Geometry check sheet. Reference: the model listing, model coordinates, mm. Give positions to 0.01 mm unless a question says otherwise; leave off trailing zeros. Loops run counter-clockwise (first coordinate to the right, second up) from the corner with the lowest first, then second, coordinate; pieces in that order, holes last. Notation, with made-up numbers: (41, -19) -> (63, -19) arc R18 cw to (63, -5) -> close; hole circle Ø8 at (36, 7.5). An arc over 180 degrees is marked (long way). Answer as a JSON object with one key per item and string values.
from build123d import *

# Parameters (mm, degrees)
SKETCH1_W           = 228.6
SKETCH1_H           = 228.6
BOSS_EXTRUDE1_DEPTH = 5.08
CUT_EXTRUDE2_REACH  = 325.329
SKETCH9_W           = 5.08
SKETCH9_H           = 12.7
SKETCH9_H_2         = 50.8
CUT_EXTRUDE7_START  = -5.08
CUT_EXTRUDE7_DEPTH  = 5.08
CUT_EXTRUDE5_REACH  = 325.329
SKETCH13_R          = 1.7
CUT_EXTRUDE6_REACH  = 325.329
SKETCH16_W          = 5.08
SKETCH16_H          = 12.7
CUT_EXTRUDE8_DEPTH  = 324.329130287
SKETCH17_W          = 20.32
SKETCH17_H          = 5.08
CUT_EXTRUDE9_DEPTH  = 324.329130287
CUT_EXTRUDE10_REACH = 325.329
SKETCH18_R          = 31.75
CUT_EXTRUDE11_REACH = 325.329
SKETCH19_W          = 20.828
SKETCH19_H          = 12.065


# Read off the part's stored shape, not the designer's step: Cut-Extrude7
with BuildPart() as part:
    # Sketch1 → Boss-Extrude1 (new body)
    with BuildSketch(Plane(origin=(0, 0, 0), x_dir=(1, 0, 0), z_dir=(0, 1, 0))):
        with Locations((114.3, 114.3)):
            Rectangle(SKETCH1_W, SKETCH1_H)
    extrude(amount=BOSS_EXTRUDE1_DEPTH)

    # Sketch9 → Cut-Extrude2 (cut, up to next)
    with BuildSketch(Plane(origin=(0, 5.08, 0), x_dir=(1, 0, 0), z_dir=(0, 1, 0)), mode=Mode.PRIVATE) as cut_extrude2_sk1:
        with Locations((27.94, 57.15)):
            Rectangle(SKETCH9_W, SKETCH9_H)
    cut_extrude2_tool1 = extrude(cut_extrude2_sk1.sketch, amount=-CUT_EXTRUDE2_REACH, mode=Mode.PRIVATE) & part.part
    # Sketch9 → Cut-Extrude2 (cut, up to next)
    with BuildSketch(Plane(origin=(0, 5.08, 0), x_dir=(1, 0, 0), z_dir=(0, 1, 0)), mode=Mode.PRIVATE) as cut_extrude2_sk2:
        with Locations((27.94, 171.45)):
            Rectangle(SKETCH9_W, SKETCH9_H)
    cut_extrude2_tool2 = extrude(cut_extrude2_sk2.sketch, amount=-CUT_EXTRUDE2_REACH, mode=Mode.PRIVATE) & part.part
    # Sketch9 → Cut-Extrude2 (cut, up to next)
    with BuildSketch(Plane(origin=(0, 5.08, 0), x_dir=(1, 0, 0), z_dir=(0, 1, 0)), mode=Mode.PRIVATE) as cut_extrude2_sk3:
        with Locations((27.94, 114.3)):
            Rectangle(SKETCH9_W, SKETCH9_H_2)
    cut_extrude2_tool3 = extrude(cut_extrude2_sk3.sketch, amount=-CUT_EXTRUDE2_REACH, mode=Mode.PRIVATE) & part.part
    # Sketch9 → Cut-Extrude2 (cut, up to next)
    with BuildSketch(Plane(origin=(0, 5.08, 0), x_dir=(1, 0, 0), z_dir=(0, 1, 0)), mode=Mode.PRIVATE) as cut_extrude2_sk4:
        with Locations((200.66, 57.15)):
            Rectangle(SKETCH9_W, SKETCH9_H)
    cut_extrude2_tool4 = extrude(cut_extrude2_sk4.sketch, amount=-CUT_EXTRUDE2_REACH, mode=Mode.PRIVATE) & part.part
    # Sketch9 → Cut-Extrude2 (cut, up to next)
    with BuildSketch(Plane(origin=(0, 5.08, 0), x_dir=(1, 0, 0), z_dir=(0, 1, 0)), mode=Mode.PRIVATE) as cut_extrude2_sk5:
        with Locations((200.66, 171.45)):
            Rectangle(SKETCH9_W, SKETCH9_H)
    cut_extrude2_tool5 = extrude(cut_extrude2_sk5.sketch, amount=-CUT_EXTRUDE2_REACH, mode=Mode.PRIVATE) & part.part
    # Sketch9 → Cut-Extrude2 (cut, up to next)
    with BuildSketch(Plane(origin=(0, 5.08, 0), x_dir=(1, 0, 0), z_dir=(0, 1, 0)), mode=Mode.PRIVATE) as cut_extrude2_sk6:
        with Locations((200.66, 114.3)):
            Rectangle(SKETCH9_W, SKETCH9_H_2)
    cut_extrude2_tool6 = extrude(cut_extrude2_sk6.sketch, amount=-CUT_EXTRUDE2_REACH, mode=Mode.PRIVATE) & part.part
    add(cut_extrude2_tool1.solids().sort_by_distance((27.94, 5.08, -57.15))[0], mode=Mode.SUBTRACT)
    add(cut_extrude2_tool2.solids().sort_by_distance((27.94, 5.08, -171.45))[0], mode=Mode.SUBTRACT)
    add(cut_extrude2_tool3.solids().sort_by_distance((27.94, 5.08, -114.3))[0], mode=Mode.SUBTRACT)
    add(cut_extrude2_tool4.solids().sort_by_distance((200.66, 5.08, -57.15))[0], mode=Mode.SUBTRACT)
    add(cut_extrude2_tool5.solids().sort_by_distance((200.66, 5.08, -171.45))[0], mode=Mode.SUBTRACT)
    add(cut_extrude2_tool6.solids().sort_by_distance((200.66, 5.08, -114.3))[0], mode=Mode.SUBTRACT)

    # Cut-Extrude7 outline → Cut-Extrude7 (cut)
    with BuildSketch(Plane.XZ.offset(CUT_EXTRUDE7_START)):
        with BuildLine():
            Line((228.6, -228.6), (228.6, -214.96095324))
            add(Edge.make_bspline(
                [(228.6, -214.96095324), (228.271324847, -215.358272881), (226.828038088, -217.01632419), (224.012197717, -219.629547006), (219.578479693, -222.607192086), (214.100555872, -225.254763581), (208.4056249, -227.207942052), (204.348403214, -228.260486737), (202.903319092, -228.6)],
                knots=[0.418523599, 0.418523599, 0.418523599, 0.418523599, 0.4375, 0.5, 0.5625, 0.625, 0.6875, 0.719133593, 0.719133593, 0.719133593, 0.719133593], degree=3))
            Line((202.903319092, -228.6), (228.6, -228.6))
        make_face()
        with BuildLine():
            ThreePointArc((164.870571061, 0), (204.294023356, -24.305976644), (228.6, -63.729428939))
            Line((228.6, -63.729428939), (228.6, 0))
            Line((228.6, 0), (164.870571061, 0))
        make_face()
        with BuildLine():
            Line((0, -228.6), (63.729428939, -228.6))
            ThreePointArc((63.729428939, -228.6), (24.305976644, -204.294023356), (0, -164.870571061))
            Line((0, -164.870571061), (0, -228.6))
        make_face()
        with BuildLine():
            ThreePointArc((0, -63.729428939), (24.305976644, -24.305976644), (63.729428939, 0))
            Line((63.729428939, 0), (0, 0))
            Line((0, 0), (0, -63.729428939))
        make_face()
    extrude(amount=CUT_EXTRUDE7_DEPTH, mode=Mode.SUBTRACT)

    # Sketch13 → Cut-Extrude5 (cut, up to next)
    with BuildSketch(Plane(origin=(0, 5.08, 0), x_dir=(1, 0, 0), z_dir=(0, 1, 0)), mode=Mode.PRIVATE) as cut_extrude5_sk1:
        with Locations(Location((26.879075631, 26.879075631, 0), (0, 0, 270))):
            Circle(SKETCH13_R)
    cut_extrude5_tool1 = extrude(cut_extrude5_sk1.sketch, amount=-CUT_EXTRUDE5_REACH, mode=Mode.PRIVATE) & part.part
    # Sketch13 → Cut-Extrude5 (cut, up to next)
    with BuildSketch(Plane(origin=(0, 5.08, 0), x_dir=(1, 0, 0), z_dir=(0, 1, 0)), mode=Mode.PRIVATE) as cut_extrude5_sk2:
        with Locations(Location((201.720924369, 201.720924369, 0), (0, 0, 270))):
            Circle(SKETCH13_R)
    cut_extrude5_tool2 = extrude(cut_extrude5_sk2.sketch, amount=-CUT_EXTRUDE5_REACH, mode=Mode.PRIVATE) & part.part
    # Sketch13 → Cut-Extrude5 (cut, up to next)
    with BuildSketch(Plane(origin=(0, 5.08, 0), x_dir=(1, 0, 0), z_dir=(0, 1, 0)), mode=Mode.PRIVATE) as cut_extrude5_sk3:
        with Locations(Location((26.879075631, 201.720924369, 0), (0, 0, 270))):
            Circle(SKETCH13_R)
    cut_extrude5_tool3 = extrude(cut_extrude5_sk3.sketch, amount=-CUT_EXTRUDE5_REACH, mode=Mode.PRIVATE) & part.part
    # Sketch13 → Cut-Extrude5 (cut, up to next)
    with BuildSketch(Plane(origin=(0, 5.08, 0), x_dir=(1, 0, 0), z_dir=(0, 1, 0)), mode=Mode.PRIVATE) as cut_extrude5_sk4:
        with Locations(Location((201.720924369, 26.879075631, 0), (0, 0, 270))):
            Circle(SKETCH13_R)
    cut_extrude5_tool4 = extrude(cut_extrude5_sk4.sketch, amount=-CUT_EXTRUDE5_REACH, mode=Mode.PRIVATE) & part.part
    add(cut_extrude5_tool1.solids().sort_by_distance((26.879076, 5.08, -26.879076))[0], mode=Mode.SUBTRACT)
    add(cut_extrude5_tool2.solids().sort_by_distance((201.720924, 5.08, -201.720924))[0], mode=Mode.SUBTRACT)
    add(cut_extrude5_tool3.solids().sort_by_distance((26.879076, 5.08, -201.720924))[0], mode=Mode.SUBTRACT)
    add(cut_extrude5_tool4.solids().sort_by_distance((201.720924, 5.08, -26.879076))[0], mode=Mode.SUBTRACT)

    # Sketch14 → Cut-Extrude6 (cut, up to next)
    with BuildSketch(Plane.XZ, mode=Mode.PRIVATE) as cut_extrude6_sk1:
        Polygon((169.959013197, -177.143218094), (162.774808301, -184.327422991), (166.366910749, -187.91952544), (173.551115646, -180.735320543), align=None)
    cut_extrude6_tool1 = extrude(cut_extrude6_sk1.sketch, amount=-CUT_EXTRUDE6_REACH, mode=Mode.PRIVATE) & part.part
    # Sketch14 → Cut-Extrude6 (cut, up to next)
    with BuildSketch(Plane.XZ, mode=Mode.PRIVATE) as cut_extrude6_sk2:
        Polygon((184.327422991, -162.774808301), (177.143218094, -169.959013197), (180.735320543, -173.551115646), (187.91952544, -166.366910749), align=None)
    cut_extrude6_tool2 = extrude(cut_extrude6_sk2.sketch, amount=-CUT_EXTRUDE6_REACH, mode=Mode.PRIVATE) & part.part
    # Sketch14 → Cut-Extrude6 (cut, up to next)
    with BuildSketch(Plane.XZ, mode=Mode.PRIVATE) as cut_extrude6_sk3:
        Polygon((65.825191699, -184.327422991), (58.640986803, -177.143218094), (55.048884354, -180.735320543), (62.233089251, -187.91952544), align=None)
    cut_extrude6_tool3 = extrude(cut_extrude6_sk3.sketch, amount=-CUT_EXTRUDE6_REACH, mode=Mode.PRIVATE) & part.part
    # Sketch14 → Cut-Extrude6 (cut, up to next)
    with BuildSketch(Plane.XZ, mode=Mode.PRIVATE) as cut_extrude6_sk4:
        Polygon((51.456781906, -169.959013197), (44.272577009, -162.774808301), (40.68047456, -166.366910749), (47.864679457, -173.551115646), align=None)
    cut_extrude6_tool4 = extrude(cut_extrude6_sk4.sketch, amount=-CUT_EXTRUDE6_REACH, mode=Mode.PRIVATE) & part.part
    # Sketch14 → Cut-Extrude6 (cut, up to next)
    with BuildSketch(Plane.XZ, mode=Mode.PRIVATE) as cut_extrude6_sk5:
        Polygon((177.143218094, -58.640986803), (184.327422991, -65.825191699), (187.91952544, -62.233089251), (180.735320543, -55.048884354), align=None)
    cut_extrude6_tool5 = extrude(cut_extrude6_sk5.sketch, amount=-CUT_EXTRUDE6_REACH, mode=Mode.PRIVATE) & part.part
    # Sketch14 → Cut-Extrude6 (cut, up to next)
    with BuildSketch(Plane.XZ, mode=Mode.PRIVATE) as cut_extrude6_sk6:
        Polygon((162.774808301, -44.272577009), (169.959013197, -51.456781906), (173.551115646, -47.864679457), (166.366910749, -40.68047456), align=None)
    cut_extrude6_tool6 = extrude(cut_extrude6_sk6.sketch, amount=-CUT_EXTRUDE6_REACH, mode=Mode.PRIVATE) & part.part
    # Sketch14 → Cut-Extrude6 (cut, up to next)
    with BuildSketch(Plane.XZ, mode=Mode.PRIVATE) as cut_extrude6_sk7:
        Polygon((44.272577009, -65.825191699), (51.456781906, -58.640986803), (47.864679457, -55.048884354), (40.68047456, -62.233089251), align=None)
    cut_extrude6_tool7 = extrude(cut_extrude6_sk7.sketch, amount=-CUT_EXTRUDE6_REACH, mode=Mode.PRIVATE) & part.part
    # Sketch14 → Cut-Extrude6 (cut, up to next)
    with BuildSketch(Plane.XZ, mode=Mode.PRIVATE) as cut_extrude6_sk8:
        Polygon((58.640986803, -51.456781906), (65.825191699, -44.272577009), (62.233089251, -40.68047456), (55.048884354, -47.864679457), align=None)
    cut_extrude6_tool8 = extrude(cut_extrude6_sk8.sketch, amount=-CUT_EXTRUDE6_REACH, mode=Mode.PRIVATE) & part.part
    add(cut_extrude6_tool1.solids().sort_by_distance((168.162962, 0, -182.531372))[0], mode=Mode.SUBTRACT)
    add(cut_extrude6_tool2.solids().sort_by_distance((182.531372, 0, -168.162962))[0], mode=Mode.SUBTRACT)
    add(cut_extrude6_tool3.solids().sort_by_distance((60.437038, 0, -182.531372))[0], mode=Mode.SUBTRACT)
    add(cut_extrude6_tool4.solids().sort_by_distance((46.068628, 0, -168.162962))[0], mode=Mode.SUBTRACT)
    add(cut_extrude6_tool5.solids().sort_by_distance((182.531372, 0, -60.437038))[0], mode=Mode.SUBTRACT)
    add(cut_extrude6_tool6.solids().sort_by_distance((168.162962, 0, -46.068628))[0], mode=Mode.SUBTRACT)
    add(cut_extrude6_tool7.solids().sort_by_distance((46.068628, 0, -60.437038))[0], mode=Mode.SUBTRACT)
    add(cut_extrude6_tool8.solids().sort_by_distance((60.437038, 0, -46.068628))[0], mode=Mode.SUBTRACT)

    # Sketch16 → Cut-Extrude8 (cut, through all)
    with BuildSketch(Plane.XZ):
        with Locations((139.7, -130.81)):
            Rectangle(SKETCH16_W, SKETCH16_H)
    extrude(amount=-CUT_EXTRUDE8_DEPTH, mode=Mode.SUBTRACT)

    # Sketch17 → Cut-Extrude9 (cut, through all)
    with BuildSketch(Plane.XZ):
        with Locations((119.38, -114.3)):
            Rectangle(SKETCH17_W, SKETCH17_H)
        with Locations((160.02, -114.3)):
            Rectangle(SKETCH17_W, SKETCH17_H)
    extrude(amount=-CUT_EXTRUDE9_DEPTH, mode=Mode.SUBTRACT)

    # Sketch18 → Cut-Extrude10 (cut, up to next)
    with BuildSketch(Plane(origin=(0, 5.08, 0), x_dir=(1, 0, 0), z_dir=(0, 1, 0)), mode=Mode.PRIVATE) as cut_extrude10_sk1:
        with Locations(Location((114.3, 63.5, 0), (0, 0, 270))):
            Circle(SKETCH18_R)
    cut_extrude10_tool1 = extrude(cut_extrude10_sk1.sketch, amount=-CUT_EXTRUDE10_REACH, mode=Mode.PRIVATE) & part.part
    add(cut_extrude10_tool1.solids().sort_by_distance((114.3, 5.08, -63.5))[0], mode=Mode.SUBTRACT)

    # Sketch19 → Cut-Extrude11 (cut, up to next)
    with BuildSketch(Plane(origin=(0, 5.08, 0), x_dir=(1, 0, 0), z_dir=(0, 1, 0)), mode=Mode.PRIVATE) as cut_extrude11_sk1:
        with Locations((171.988363225, 90.574772783)):
            Rectangle(SKETCH19_W, SKETCH19_H)
    cut_extrude11_tool1 = extrude(cut_extrude11_sk1.sketch, amount=-CUT_EXTRUDE11_REACH, mode=Mode.PRIVATE) & part.part
    add(cut_extrude11_tool1.solids().sort_by_distance((171.988363, 5.08, -90.574773))[0], mode=Mode.SUBTRACT)


solid = part.part
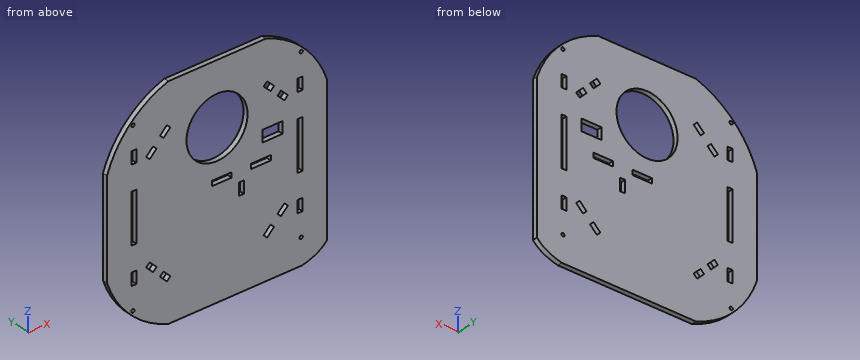
1) Depth check by flat-ended pin: P1, Ø1.5, axis at y = 3.5, z = -168.5, coming from the -X side; P2, Ø1.5, axis at x = 168, y = 3, coming from the +Z side; P3, Ø1.5, axis at x = 26.5, y = 2, coming from the +Z side; P4, Ø2, axis at x = 26.88, z = -26.88, coming from the -Y side. Enter the tip coordinate at first touch or a pass-through.
Geometry check:
{"P1": "stops at x = 1", "P2": "stops at z = -0.82", "P3": "stops at z = -21.48", "P4": "passes through"}
2) Section check D-D on y = 1.65. Count the separate pieces of the cut face and the enclosed holes in it, plus the area to 3 significant figures.
Geometry check:
{"separate pieces": "1", "enclosed holes": "23", "area": "43,100 mm2"}
3) Section check A-A on z = -120.5. Record the cut outline in (x, y), plus the area to 3 significant figures.
Geometry check:
{"outline": "(0, 0) -> (25.4, 0) -> (25.4, 5.08) -> (0, 5.08) -> close; (30.48, 0) -> (198.12, 0) -> (198.12, 5.08) -> (30.48, 5.08) -> close; (203.2, 0) -> (228.6, 0) -> (228.6, 5.08) -> (203.2, 5.08) -> close", "area": "1,110 mm2"}
4) Material ranges on line 1 along X through (y, z) = (1.2, -119.5); line 2 along X through (y, z) = (2.95, -132); line 3 along Z through (x, y) = (117, 1.35), recorded low to high. Write a range as from..to.
Geometry check:
{"line 1": "x = 0..25.4, 30.48..198.12, 203.2..228.6", "line 2": "x = 0..25.4, 30.48..137.16, 142.24..198.12, 203.2..228.6", "line 3": "z = -228.6..-116.84, -111.76..-95.13, -31.87..0"}
5) Section check B-B on x = 121. Record the cut outline in (y, z).
Geometry check:
{"outline": "(0, -228.6) -> (5.08, -228.6) -> (5.08, -116.84) -> (0, -116.84) -> close; (0, -111.76) -> (5.08, -111.76) -> (5.08, -94.54) -> (0, -94.54) -> close; (0, -32.46) -> (5.08, -32.46) -> (5.08, 0) -> (0, 0) -> close"}
6) Section check C-C on x = 21. Record the cut outline in (y, z).
Geometry check:
{"outline": "(0, -200.83) -> (5.08, -200.83) -> (5.08, -27.77) -> (0, -27.77) -> close"}
